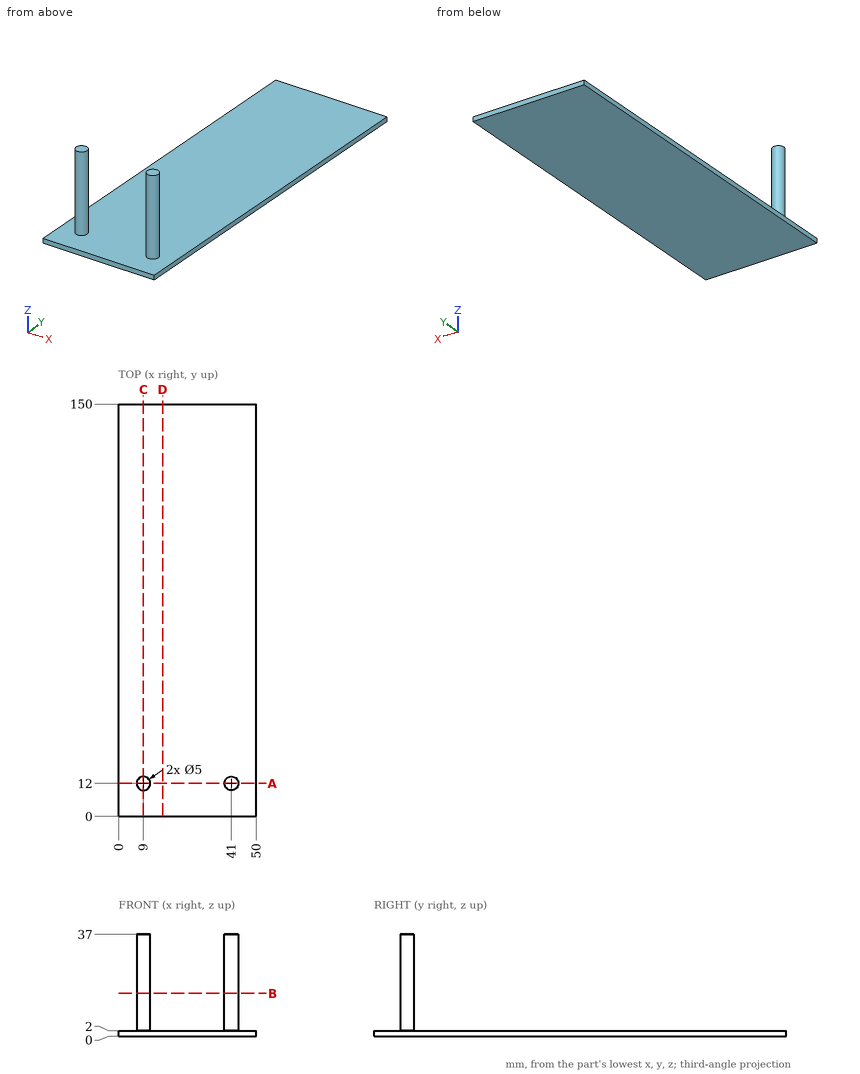
The figure shows three views and two pictorial views of one solid part (mm, origin at its lowest corner). Answer the questions. Give positions to 0.01 mm unless a question says otherwise; leave off trailing zeros. Loops run counter-clockwise (first coordinate to the right, second up) from the corner with the lowest first, then second, coordinate; pieces in that order, holes last. Notation, with made-up numbers: (50.25, 25) -> (74.25, 25) arc R12 ccw to (74.25, 35) -> close; hole circle Ø10 at (42.5, 0). An arc over 180 degrees is marked (long way). Use CSV: the item, a comma, the result in double quotes.
1. The part is cut by section D-D (x = 16). Write down the section's boundary in (y, z), then the cut area to 3 significant figures.
Found:
outline,"(0, 0) -> (150, 0) -> (150, 2) -> (0, 2) -> close"
area,"300 mm^2"
2. The part is cut by section B-B (z = 15.5). Write down the section's boundary in (x, y).
Found:
outline,"circle Ø5 at (9, 12); circle Ø5 at (41, 12)"
3. Straight lines are drawn through the part: line 1 (Z direction, x = 47, y = 19); line 2 (Y direction, x = 39, z = 11.5); line 3 (Y direction, x = 39.5, z = 30). For each, find the intervals that lie inside material, in ascending order.
Found:
line 1,"0 to 2"
line 2,"10.5 to 13.5"
line 3,"10 to 14"
4. The part is cut by section A-A (y = 12). Write down the section's boundary in (x, z).
Found:
outline,"(0, 0) -> (50, 0) -> (50, 2) -> (43.5, 2) -> (43.5, 37) -> (38.5, 37) -> (38.5, 2) -> (11.5, 2) -> (11.5, 37) -> (6.5, 37) -> (6.5, 2) -> (0, 2) -> close"
5. The part is cut by section C-C (x = 9). Write down the section's boundary in (y, z).
Found:
outline,"(0, 0) -> (150, 0) -> (150, 2) -> (14.5, 2) -> (14.5, 37) -> (9.5, 37) -> (9.5, 2) -> (0, 2) -> close"
6. A flat-ended cylindrical pin translates along its axis: pin 1 Ø6 at (x, y) = (20, 127.5) entering from -Z. Find the tip coordinate at first contact, or state that the pin passes through.
Found:
pin 1,"z = 0"
